```python
from build123d import *

# Parameters (mm, degrees)
F0_W      = 685.8
F0_H      = 25.4
F1_DEPTH  = 304.8
F2_W      = 25.4
F2_H      = 304.8
F3_DEPTH  = 304.8
F4_DEPTH  = 304.8
F5_W      = 25.4
F5_H      = 304.8
F6_DEPTH  = 660.4
F7_W      = 655.32
F7_H      = 5.08
F7_W_2    = 5.08
F7_H_2    = 299.72
F7_W_3    = 2.54
F8_DEPTH  = 5.08
F9_W      = 63.5
F9_H      = 63.5
F10_DEPTH = 25.4


with BuildPart() as f1:
    # F0 (on Top) → F1 (new body)
    with BuildSketch(Plane.XY):
        with Locations((342.9, -12.7)):
            Rectangle(F0_W, F0_H)
    extrude(amount=F1_DEPTH)

    # F2 (on face) → F3 (join)
    with BuildSketch(Plane.XZ.offset(25.4)):
        with Locations((673.1, 152.4)):
            Rectangle(F2_W, F2_H)
    extrude(amount=F3_DEPTH)

    # F2 (on face) → F4 (join)
    with BuildSketch(Plane.XZ.offset(25.4)):
        with Locations((12.7, 152.4)):
            Rectangle(F2_W, F2_H)
    extrude(amount=F4_DEPTH)

    # F5 (on face) → F6 (join)
    with BuildSketch(Plane.YZ.offset(25.4)):
        with Locations((-317.5, 152.4)):
            Rectangle(F5_W, F5_H)
    extrude(amount=F6_DEPTH)

    # F7 (on face) → F8 (cut)
    with BuildSketch(Plane.XY.offset(304.8)):
        with Locations((342.9, -12.7)):
            Rectangle(F7_W, F7_H)
        Polygon((15.24, -10.16), (12.7, -10.16), (10.16, -10.16), (10.16, -15.24), (15.24, -15.24), align=None)
        with Locations((12.7, -165.1)):
            Rectangle(F7_W_2, F7_H_2)
        with Locations((12.7, -317.5)):
            Rectangle(F7_W_2, F7_H)
        with Locations((342.9, -317.5)):
            Rectangle(F7_W, F7_H)
        with Locations((673.1, -317.5)):
            Rectangle(F7_W_2, F7_H)
        Polygon((675.64, -10.16), (673.1, -10.16), (673.1, -15.24), (670.56, -15.24), (670.56, -314.96), (675.64, -314.96), align=None)
        with Locations((671.83, -12.7)):
            Rectangle(F7_W_3, F7_H)
    extrude(amount=-F8_DEPTH, mode=Mode.SUBTRACT)

    # F9 (on face) → F10 (cut)
    with BuildSketch(Plane(origin=(0, 0, 0), x_dir=(1, 0, 0), z_dir=(0, 0, -1))):
        with Locations((654.05, 31.75)):
            Rectangle(F9_W, F9_H)
        with Locations((654.05, 298.45)):
            Rectangle(F9_W, F9_H)
        with Locations((31.75, 298.45)):
            Rectangle(F9_W, F9_H)
        with Locations((31.75, 31.75)):
            Rectangle(F9_W, F9_H)
    extrude(amount=-F10_DEPTH, mode=Mode.SUBTRACT)


solid = f1.part
```
The listing builds one solid part. Answer for the finished solid, in the listing's coordinates (mm). A direction names the side the tool comes from. Give positions to 0.01 mm unless a question says otherwise; leave off trailing zeros. Order: outer loops, then holes, each group sorted by start corner. A loop starts at its lowest first (then second) coordinate and runs counter-clockwise, first axis right, second up.
1) For faces 4 (the face through (338, -304.8, 150)), 5 (the face through (63.5, -13, 13)), 6 (the face through (661, -25, 25.4)), 7 (the face through (24, -306, 25.4)), 8 (the face through (13, -63.5, 13)), determine the directions among +Z, -Z, +X, -X, +Y, -Y from which every point of the face is accessible in a straight line to the end or side of a thin tool.
Reported:
face 4: +Z, -Z
face 5: -Z, -X, +Y, -Y
face 6: -Z, +X, +Y
face 7: -Z, -X, -Y
face 8: -Z, +X, -X, +Y
2) Find section C-C on z = 220. Write down the section's boundary in (x, y), then the cut area to 3 significant figures.
Reported:
outline: (0, -330.2) - (685.8, -330.2) - (685.8, 0) - (0, 0) - close; hole (25.4, -304.8) - (660.4, -304.8) - (660.4, -25.4) - (25.4, -25.4) - close
area: 49,000 mm2
3) Determine the mould class of faces 1 (the face through (622.3, -13, 13)), 2 (the face through (341, -325, 304.8)), 3 (the face through (341, -15, 299.72)) for opening direction X: pulls with the +X half, pulls with the -X half, needs draft (parallel to the pull), parting line crosses it, or undercut.
Reported:
face 1: pulls with the +X half
face 2: needs draft
face 3: undercut
4) Find section B-B on x = 272.5. Write down the section's boundary in (y, z), then the cut area to 3 significant figures.
Reported:
outline: (-330.2, 0) - (-304.8, 0) - (-304.8, 304.8) - (-314.96, 304.8) - (-314.96, 299.72) - (-320.04, 299.72) - (-320.04, 304.8) - (-330.2, 304.8) - close; (-25.4, 0) - (0, 0) - (0, 304.8) - (-10.16, 304.8) - (-10.16, 299.72) - (-15.24, 299.72) - (-15.24, 304.8) - (-25.4, 304.8) - close
area: 15,400 mm2
5) Find section A-A on y = -210. Write down the section's boundary in (x, z).
Reported:
outline: (0, 0) - (25.4, 0) - (25.4, 304.8) - (15.24, 304.8) - (15.24, 299.72) - (10.16, 299.72) - (10.16, 304.8) - (0, 304.8) - close; (660.4, 0) - (685.8, 0) - (685.8, 304.8) - (675.64, 304.8) - (675.64, 299.72) - (670.56, 299.72) - (670.56, 304.8) - (660.4, 304.8) - close
6) Given P1, Ø20.5, axis at x = 8, z = 7.5, coming from the -Y side; P2, Ø12.5, axis at y = -322, z = 18.5, coming from the +X side; P3, Ø19, axis at x = 654.5, y = -289, coming from the -Z side, each flat-ended and moving along its own axis, determine where each tip first touches the part or whether it passes through.
Reported:
P1: stops at y = -266.7
P2: stops at x = 622.3
P3: stops at z = 25.4
7) Consider line 1 along Y through (x, z) = (457.5, 71); line 2 along X through (y, z) = (-159.5, 29). Determine where each line is inside the solid, lowest interval first.
Reported:
line 1: y = -330.2 to -304.8, -25.4 to 0
line 2: x = 0 to 25.4, 660.4 to 685.8
